Study the drawing (mm; zero at the part's minimum x, y, z) and answer. A direction names the side the tool comes from. Coordinates: 2 decimals unless noted, no trailing zeros. Order: outer loops, then holes, each group sorted by start corner. A loop starts at its lowest first (then second) coordinate and runs counter-clockwise, first axis right, second up.
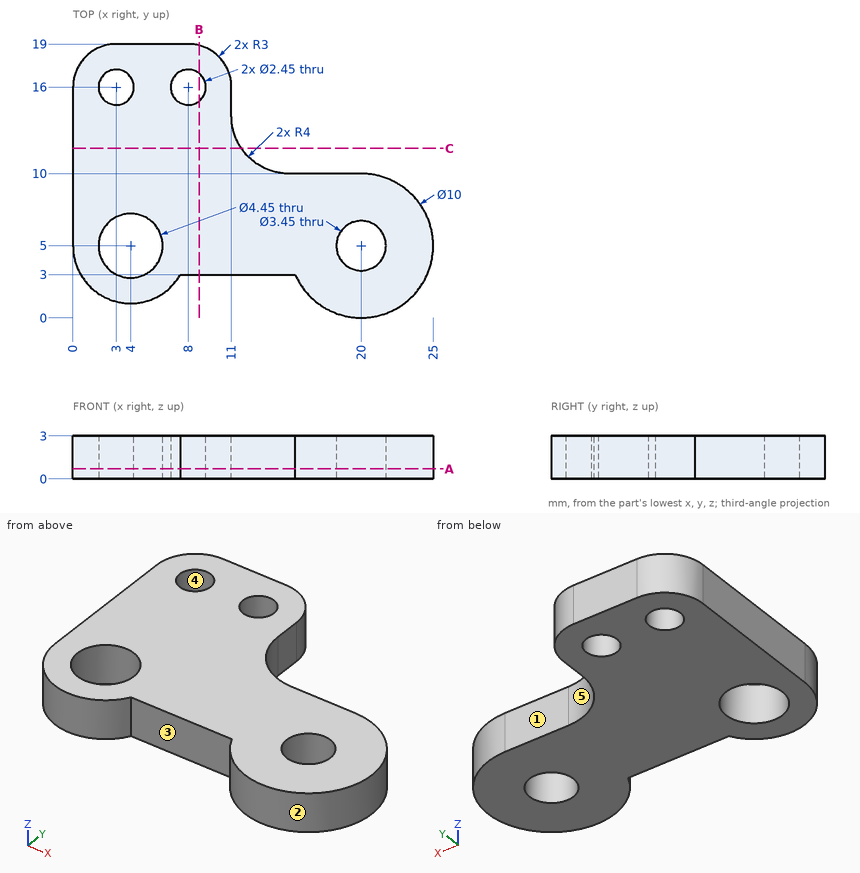
(1) The mould has two halves that part along Y. Classify the marked faces 3, 4 and 5: released by +Y, released by -Y, zero draft, split by the parting line, or undercut.
(2) Find section C-C (y = 11.75). Write down the section's boundary in (x, z), and give its area (3 significant figures).
(3) For the marked faces 1 and 2, determine the directions among +Z, -Z, +X, -X, +Y, -Y from which every point of the face is accessible in a straight line to the end or side of a thin tool.
(4) Consider line 1 (X direction, y = 4.25, z = 0.25); line 2 (Y direction, x = 8, z = 0.95) (3 decimals); line 3 (Y direction, x = 20, z = 2.05) (3 decimals). Determine where each line is inside the solid, lowest interval first.
(5) Find section B-B (x = 8.75). Write down the section's boundary in (y, z), and give its area (3 significant figures).
(6) Find section A-A (z = 0.7). Write down the section's boundary in (x, y) (3 decimals).
(7) Each of these flat-tipped pins is pushed along its axis until it touches: pin 1 Ø1.5 at (x, z) = (10, 1) entering from +Y; pin 2 Ø1 at (x, z) = (13.5, 2.5) entering from +Y; pin 3 Ø2 at (x, y) = (20, 5) entering from -Z; pin 4 Ø1 at (y, z) = (15, 1) entering from +X. Where does it stop, or does it pass through?
Findings below:
1. face 3: released by -Y
1. face 4: undercut
1. face 5: released by +Y
2. outline: (0, 0) - (11.69, 0) - (11.69, 3) - (0, 3) - close
2. area: 35.1 mm2
3. face 1: +Z, -Z, +X, +Y
3. face 2: +Z, -Z
4. line 1: x = 0.07 to 1.91, 6.09 to 18.45, 21.55 to 24.94
4. line 2: y = 3 to 14.775, 17.225 to 19
4. line 3: y = 0 to 3.275, 6.725 to 10
5. outline: (3, 0) - (15.03, 0) - (15.03, 3) - (3, 3) - close; (16.97, 0) - (18.9, 0) - (18.9, 3) - (16.97, 3) - close
5. area: 41.9 mm2
6. outline: (0, 5) arc R4 ccw to (7.464, 3) - (15.417, 3) arc R5 ccw (long way) to (20, 10) - (15, 10) arc R4 cw to (11, 14) - (11, 16) arc R3 ccw to (8, 19) - (3, 19) arc R3 ccw to (0, 16) - close; hole circle Ø4.45 at (4, 5); hole circle Ø2.45 at (3, 16); hole circle Ø2.45 at (8, 16); hole circle Ø3.45 at (20, 5)
7. pin 1: stops at y = 18.73
7. pin 2: stops at y = 10.54
7. pin 3: passes through
7. pin 4: stops at x = 11
